Work out the finished part from the listing and answer in its coordinate system (mm). A direction names the side the tool comes from. Give positions to 0.01 mm unless a question says otherwise; leave off trailing zeros. Loops run counter-clockwise (first coordinate to the right, second up) from the corner with the lowest first, then second, coordinate; pieces in that order, holes last. Notation, with made-up numbers: (17.5, 71) - (73.5, 71) arc R21 cw to (73.5, 100) - close; hole circle Ø6 at (-17.75, 76). An arc over 180 degrees is marked (long way). One line per item, written item: value.
from build123d import *

# Parameters (mm, degrees)
SKETCH1_R                = 16
SKETCH1_R_2              = 11
BOSS_EXTRUDE1_DEPTH      = 20
SKETCH2_R                = 16
BOSS_EXTRUDE2_DEPTH      = 2
BOSS_EXTRUDE3_DEPTH      = 16
BOSS_EXTRUDE3_DEPTH_BACK = 16
CUT_EXTRUDE1_DEPTH       = 30.002175046
BOSS_EXTRUDE4_REACH      = 31.002
SKETCH5_R                = 16
SKETCH6_R                = 2.6
CUT_EXTRUDE3_DEPTH       = 29.757190977


with BuildPart() as part:
    # Sketch1 → Boss-Extrude1 (new body)
    with BuildSketch(Plane.XY):
        Circle(SKETCH1_R)
        Circle(SKETCH1_R_2, mode=Mode.SUBTRACT)
    extrude(amount=BOSS_EXTRUDE1_DEPTH)

    # Sketch2 → Boss-Extrude2 (add)
    with BuildSketch(Plane(origin=(0, 0, 0), x_dir=(-1, 0, 0), z_dir=(0, 0, -1))):
        Circle(SKETCH2_R)
    extrude(amount=BOSS_EXTRUDE2_DEPTH)

    # Sketch3 → Boss-Extrude3 (add, two sides)
    with BuildSketch(Plane(origin=(0, 0, 0), x_dir=(0, 0, -1), z_dir=(1, 0, 0))) as boss_extrude3_sk:
        Polygon((31.002175046, 25.419398483), (26.906414824, 28.287280664), (18.302768279, 16), (2, -7.282766022), (2, -16), align=None)
    extrude(amount=BOSS_EXTRUDE3_DEPTH)
    extrude(boss_extrude3_sk.sketch, amount=-BOSS_EXTRUDE3_DEPTH_BACK)

    # Sketch4 → Cut-Extrude1 (cut, through all)
    with BuildSketch(Plane(origin=(0, 0, -2), x_dir=(-1, 0, 0), z_dir=(0, 0, -1))):
        with BuildLine():
            Line((34.266518051, 0), (16, 0))
            ThreePointArc((16, 0), (15.555436181, -3.745451268), (14.24644935, -7.282766022))
            ThreePointArc((14.24644935, -7.282766022), (0, -16), (-14.24644935, -7.282766022))
            ThreePointArc((-14.24644935, -7.282766022), (-15.555436181, -3.745451268), (-16, 0))
            Line((-16, 0), (-34.430612934, 0))
            Line((-34.430612934, 0), (-36.46308972, -20.488677285))
            Line((-36.46308972, -20.488677285), (32.179774964, -27.298049462))
            Line((32.179774964, -27.298049462), (34.266518051, 0))
        make_face()
    extrude(amount=CUT_EXTRUDE1_DEPTH, mode=Mode.SUBTRACT)

    # Sketch5 → Boss-Extrude4 (add, up to next)
    with BuildSketch(Plane(origin=(0, 0, -2), x_dir=(-1, 0, 0), z_dir=(0, 0, -1)), mode=Mode.PRIVATE) as boss_extrude4_sk1:
        Circle(SKETCH5_R)
    boss_extrude4_tool1 = extrude(boss_extrude4_sk1.sketch, amount=BOSS_EXTRUDE4_REACH, mode=Mode.PRIVATE) - part.part
    add(boss_extrude4_tool1.solids().sort_by_distance((0, 0, -2))[0])

    # Sketch6 → Cut-Extrude3 (cut, through all)
    with BuildSketch(Plane(origin=(0, -3.335649292, -4.763800888), x_dir=(1, 0, 0), z_dir=(0, 0.573576436, 0.819152044))):
        with Locations((0, 31.104469313)):
            Circle(SKETCH6_R)
    extrude(amount=-CUT_EXTRUDE3_DEPTH, mode=Mode.SUBTRACT)


solid = part.part
1. Section D-D (x = -8.5) is taken. Write down the section's boundary in (y, z).
Output:
outline: (-13.56, -3.71) - (25.42, -31) - (28.29, -26.91) - (13.56, -16.59) - (13.56, 20) - (6.98, 20) - (6.98, 0) - (-6.98, 0) - (-6.98, 20) - (-13.56, 20) - close
2. Section A-A (z = 16) is taken. Write down the section's boundary in (x, y).
Output:
outline: circle Ø32 at (0, 0); hole circle Ø22 at (0, 0)
3. Flat-ended cylindrical pins translate along their axes: pin 1 Ø17.5 at (x, y) = (0, 0) entering from -Z; pin 2 Ø3 at (x, z) = (-2.5, -6.5) entering from -Y; pin 3 Ø8 at (x, y) = (-6, -7.5) entering from -Z. Find the tip coordinate at first contact, or state that the pin passes through.
Output:
pin 1: stops at z = -19.33
pin 2: stops at y = -11.72
pin 3: stops at z = -10.75
4. Section B-B (x = 1.5) is taken. Write down the section's boundary in (y, z).
Output:
outline: (-15.93, -2.05) - (17.54, -25.48) - (20.4, -21.39) - (15.93, -18.25) - (15.93, 20) - (10.9, 20) - (10.9, 0) - (-10.9, 0) - (-10.9, 20) - (-15.93, 20) - close; (21.02, -27.92) - (25.42, -31) - (28.29, -26.91) - (23.88, -23.82) - close
5. Find the intervals of material crossed by line 1 along Y through (x, z) = (0, 7); line 2 along Y through (x, z) = (-12, -10); line 3 along Z through (x, y) = (-12, -3.5), in increasing order.
Output:
line 1: y = -16 to -11, 11 to 16
line 2: y = -4.57 to 10.58
line 3: z = -10.75 to 20
6. For faces 5 (the cylindrical face through (-2.38, -10.74, 9.86)), 6 (the flat face through (-16, 14, -20)), determine the directions among +Z, -Z, +X, -X, +Y, -Y from which every point of the face is accessible in a straight line to the end or side of a thin tool.
Output:
face 5: +Z
face 6: +Z, -Z, -X, +Y, -Y
7. The mould has two halves that part along X. Classify faces 1 (the flat face through (0, 0, 0)), 2 (the flat face through (3, 11, 20)), 3 (the flat face through (16, 14, -20)), 4 (the cylindrical face through (-0.56, 18.65, -23.17)): released by +X, released by -X, zero draft, split by the parting line, or undercut.
Output:
face 1: undercut
face 2: zero draft
face 3: released by +X
face 4: undercut
8. Section C-C (y = 5.5) is taken. Write down the section's boundary in (x, z), and give its area (3 significant figures).
Output:
outline: (-16, -17.05) - (16, -17.05) - (16, -10.95) - (15.02, -10.95) - (15.02, 20) - (9.53, 20) - (9.53, 0) - (-9.53, 0) - (-9.53, 20) - (-15.02, 20) - (-15.02, -10.95) - (-16, -10.95) - close
area: 744 mm²
